Input: part model. Units: mm. Frame: model coordinates. A direction names the side the tool comes from. Round coordinates to 2 decimals unless told otherwise and drop trailing zeros. Order: outer loops, then holes, each group sorted by start corner. A loop starts at its lowest first (then second) coordinate and runs counter-clockwise, first axis right, second up. Notation, with made-up numbers: (68.25, 4) -> (96.25, 4) arc R19 ccw to (96.25, 21) -> close; hole circle Ø9 at (-26, 15). An arc over 180 degrees is marked (long way). Use a Markdown table: item, result.
from build123d import *

# Parameters (mm, degrees)
SKETCH_2_R               = 120
EXTRUDE_1_DEPTH          = 15
CUT_EXTRUDE_1_DEPTH      = 171.367250374
CUT_EXTRUDE_1_DEPTH_BACK = 171.367250374
SKETCH_3_R               = 7.5
SKETCH_4_R               = 15
EXTRUDE_2_DEPTH          = 119
SKETCH_5_R               = 20
EXTRUDE_3_DEPTH          = 72.58
SKETCH_7_W               = 15
SKETCH_7_H               = 90.968276451
CUT_EXTRUDE_3_DEPTH      = 60
CUT_EXTRUDE_4_DEPTH      = 222.970934419
CUT_EXTRUDE_4_DEPTH_BACK = 222.970934419
SKETCH_8_R               = 7.5
CUT_EXTRUDE_5_DEPTH      = 222.970934419
CUT_EXTRUDE_5_DEPTH_BACK = 222.970934419
SKETCH_9_R               = 7.5
CUT_EXTRUDE_6_DEPTH      = 221.481858664
CUT_EXTRUDE_6_DEPTH_BACK = 221.481858664
SKETCH_10_R              = 7.5
SKETCH_11_R              = 22.5
EXTRUDE_4_DEPTH          = 5
SKETCH_12_R              = 1.5
CUT_EXTRUDE_7_DEPTH      = 10


with BuildPart() as part:
    # 草图2 → 凸台-拉伸1 (new body)
    with BuildSketch(Plane(origin=(0, 0, 0), x_dir=(0, 0, -1), z_dir=(1, 0, 0))):
        Circle(SKETCH_2_R)
    extrude(amount=EXTRUDE_1_DEPTH)

    # 草图3 → 切除-拉伸1 (cut, two sides: drawn at the far end of the back side and taken through both)
    with BuildSketch(Plane.ZY.offset(-CUT_EXTRUDE_1_DEPTH_BACK)):
        with Locations((0, 29.25)):
            Circle(SKETCH_3_R)
        with Locations((25.331243061, -14.625)):
            Circle(SKETCH_3_R)
        with Locations((-25.331243061, -14.625)):
            Circle(SKETCH_3_R)
    extrude(amount=CUT_EXTRUDE_1_DEPTH + CUT_EXTRUDE_1_DEPTH_BACK, mode=Mode.SUBTRACT)

    # 草图4 → 凸台-拉伸2 (add)
    with BuildSketch(Plane(origin=(15, 0, 0), x_dir=(0, 0, -1), z_dir=(1, 0, 0))):
        with Locations((0, 80)):
            Circle(SKETCH_4_R)
        with Locations((80, 0)):
            Circle(SKETCH_4_R)
        with Locations((0, -80)):
            Circle(SKETCH_4_R)
        with Locations((-80, 0)):
            Circle(SKETCH_4_R)
    extrude(amount=EXTRUDE_2_DEPTH)

    # 草图5 → 凸台-拉伸3 (add)
    with BuildSketch(Plane.ZY):
        with Locations(Location((0, 90, 0), (0, 0, 180))):
            Circle(SKETCH_5_R)
        with Locations(Location((77.942286341, -45, 0), (0, 0, 180))):
            Circle(SKETCH_5_R)
        with Locations(Location((-77.942286341, -45, 0), (0, 0, 180))):
            Circle(SKETCH_5_R)
    extrude(amount=EXTRUDE_3_DEPTH)

    # 草图7 → 切除-拉伸3 (cut)
    with BuildSketch(Plane.ZY.offset(72.58)):
        Polygon((51.844496006, -38.592687763), (130.625334351, -84.076825989), (138.125334351, -71.086444932), (59.344496006, -25.602306706), align=None)
        Polygon((-51.844496006, -38.592687763), (-59.344496006, -25.602306706), (-138.125334351, -71.086444932), (-130.625334351, -84.076825989), align=None)
        with Locations((0, 109.679132694)):
            Rectangle(SKETCH_7_W, SKETCH_7_H)
    extrude(amount=-CUT_EXTRUDE_3_DEPTH, mode=Mode.SUBTRACT)

    # 草图8 → 切除-拉伸4 (cut, two sides: drawn at the far end of the back side and taken through both)
    with BuildSketch(Plane(origin=(0, 6.495190528, 3.75), x_dir=(1, 0, 0), z_dir=(0, -0.8660254037844389, -0.4999999999999997)).offset(-CUT_EXTRUDE_4_DEPTH_BACK)):
        with Locations(Location((-42.58, 90, 0), (0, 0, 270))):
            Circle(SKETCH_8_R)
    extrude(amount=CUT_EXTRUDE_4_DEPTH + CUT_EXTRUDE_4_DEPTH_BACK, mode=Mode.SUBTRACT)

    # 草图9 → 切除-拉伸5 (cut, two sides: drawn at the far end of the back side and taken through both)
    with BuildSketch(Plane(origin=(0, -6.495190528, 3.75), x_dir=(1, 0, 0), z_dir=(0, 0.8660254037844386, -0.5000000000000003)).offset(-CUT_EXTRUDE_5_DEPTH_BACK)):
        with Locations(Location((-42.58, 90, 0), (0, 0, 270))):
            Circle(SKETCH_9_R)
    extrude(amount=CUT_EXTRUDE_5_DEPTH + CUT_EXTRUDE_5_DEPTH_BACK, mode=Mode.SUBTRACT)

    # 草图10 → 切除-拉伸6 (cut, two sides: drawn at the far end of the back side and taken through both)
    with BuildSketch(Plane.XY.offset(-7.5).offset(-CUT_EXTRUDE_6_DEPTH_BACK)):
        with Locations((-42.58, 90)):
            Circle(SKETCH_10_R)
    extrude(amount=CUT_EXTRUDE_6_DEPTH + CUT_EXTRUDE_6_DEPTH_BACK, mode=Mode.SUBTRACT)

    # 草图11 → 凸台-拉伸4 (add)
    with BuildSketch(Plane(origin=(134, 0, 0), x_dir=(0, 0, -1), z_dir=(1, 0, 0))):
        with Locations((-80, 0)):
            Circle(SKETCH_11_R)
        with Locations((0, 80)):
            Circle(SKETCH_11_R)
        with Locations((80, 0)):
            Circle(SKETCH_11_R)
        with Locations((0, -80)):
            Circle(SKETCH_11_R)
    extrude(amount=EXTRUDE_4_DEPTH)

    # 草图12 → 切除-拉伸7 (cut)
    with BuildSketch(Plane(origin=(139, 0, 0), x_dir=(0, 0, -1), z_dir=(1, 0, 0))):
        with Locations((-60, 0)):
            Circle(SKETCH_12_R)
        with Locations((-80, -20)):
            Circle(SKETCH_12_R)
        with Locations((-100, 0)):
            Circle(SKETCH_12_R)
        with Locations((-80, 20)):
            Circle(SKETCH_12_R)
        with Locations((0, 60)):
            Circle(SKETCH_12_R)
        with Locations((60, 0)):
            Circle(SKETCH_12_R)
        with Locations((0, -60)):
            Circle(SKETCH_12_R)
        with Locations((20, 80)):
            Circle(SKETCH_12_R)
        with Locations((80, -20)):
            Circle(SKETCH_12_R)
        with Locations((-20, -80)):
            Circle(SKETCH_12_R)
        with Locations((0, 100)):
            Circle(SKETCH_12_R)
        with Locations((100, 0)):
            Circle(SKETCH_12_R)
        with Locations((0, -100)):
            Circle(SKETCH_12_R)
        with Locations((-20, 80)):
            Circle(SKETCH_12_R)
        with Locations((80, 20)):
            Circle(SKETCH_12_R)
        with Locations((20, -80)):
            Circle(SKETCH_12_R)
    extrude(amount=-CUT_EXTRUDE_7_DEPTH, mode=Mode.SUBTRACT)


solid = part.part
1) Cut plane A-A on x = -19. Return loops of the section in (y, z), and give its area (3 significant figures).
Results found:
| item | result |
|---|---|
| outline | (-60.77, -90.25) -> (-42.22, -58.14) arc R20 ccw to start; (-60.77, 90.25) arc R20 ccw to (-42.22, 58.14) -> close; (-47.78, -97.75) arc R20 ccw to (-29.23, -65.64) -> close; (-47.78, 97.75) -> (-29.23, 65.64) arc R20 ccw to start; (71.46, -7.5) arc R20 ccw to (108.54, -7.5) -> close; (71.46, 7.5) -> (108.54, 7.5) arc R20 ccw to start |
| area | 2,010 mm² |
2) Set-up query: faces 4 (the cylindrical face through (136.46, 0.99, -57.52)), 5 (the flat face through (0, 2, 2)), 6 (the cylindrical face through (73.667, 65.357, 3.252)). Return all of +Z, -Z, +X, -X, +Y, -Y with unobstructed straight access to the full face (end or side cutting, diameter ignored); none if empty.
Results found:
| item | result |
|---|---|
| face 4 | +X |
| face 5 | -X |
| face 6 | none |
3) Pin query (flat end, axial travel): pin 1 Ø2 at (x, z) = (-29.5, 14) entering from -Y; pin 2 Ø6 at (y, z) = (35, 45) entering from +X; pin 3 Ø17 at (x, y) = (-42.58, 90) entering from -Z; pin 4 Ø9 at (y, z) = (-14.62, -25.33) entering from +X. Return the tip coordinate at first contact, or that it passes through.
Results found:
| item | result |
|---|---|
| pin 1 | stops at y = 74.8 |
| pin 2 | stops at x = 15 |
| pin 3 | stops at z = -20 |
| pin 4 | passes through |
4) Cut plane D-D on z = 37.5. Return loops of the section in (x, y), and give its area (3 significant figures).
Results found:
| item | result |
|---|---|
| outline | (0, -113.99) -> (15, -113.99) -> (15, 113.99) -> (0, 113.99) -> close |
| area | 3,420 mm² |
5) Cut plane C-C on z = -29. Return loops of the section in (x, y).
Results found:
| item | result |
|---|---|
| outline | (0, -116.44) -> (15, -116.44) -> (15, -21.17) -> (0, -21.17) -> close; (0, -8.08) -> (15, -8.08) -> (15, 116.44) -> (0, 116.44) -> close |
6) Pull-direction query (Y, two-part tool) for faces 1 (the cylindrical face through (73.667, 4.506, 65.693)), 2 (the flat face through (-50, 86, 7.5)), 3 (the flat face through (134, -85, -15)); classes: +Y half, -Y half, draft (parallel to the pull), parting line (faces both ways), or undercut.
Results found:
| item | result |
|---|---|
| face 1 | parting line |
| face 2 | draft |
| face 3 | undercut |
7) Cut plane B-B on x = 56. Return loops of the section in (y, z).
Results found:
| item | result |
|---|---|
| outline | circle Ø30 at (-80, 0); circle Ø30 at (0, -80); circle Ø30 at (0, 80); circle Ø30 at (80, 0) |
8) Line query: L1, parallel to X at y = 90, z = -11.75; L2, parallel to X at y = -98, z = -5.5; L3, parallel to X at y = -102, z = 28. Output: solid intervals per line, ascending. Write a range as [from, to].
Results found:
| item | result |
|---|---|
| L1 | x = [-72.58, -50.08], [-35.08, 15], [134, 139] |
| L2 | x = [0, 15], [134, 139] |
| L3 | x = [0, 15] |
